Input: dimensioned drawing with shaded views. Units: mm. Origin: part minimum x, y, z. Coordinates: 2 decimals unless noted, no trailing zeros. Write each loop counter-clockwise with the first axis right and the second up, starting at its lowest first coordinate (ties: lowest second). Pieces come first, ordered by that corner, then holes. Notation, with made-up numbers: (35.5, 40) -> (73.5, 40) arc R23 ccw to (73.5, 69) -> close; hole circle Ø7 at (-31, -26.5). An arc over 180 degrees is marked (long way). One line per item, written item: value. Start each with the question number.
1. Section query A-A, the plane x = 7.5. Output: boundary loops of the cut face in (y, z).
2. Section query C-C, the plane z = 9.75. Output: boundary loops of the cut face in (x, y).
3. Line query: line 1 (Y direction, x = 7.5, z = 7); line 2 (Y direction, x = 10.5, z = 6.25); line 3 (X direction, y = 27, z = 5.25). Output: solid intervals per line, ascending.
4. Mould query, pull axis Y, two halves, no side actions, for the marked faces 1, 2 and 3. Classes: released by +Y, released by -Y, zero draft, split by the parting line, or undercut.
5. First-contact query: P1, Ø3, axis at x = 2.5, y = 25.5, coming from the -Z side; P2, Ø9, axis at x = 7.5, y = 30, coming from the -Z side. Flat tips, straight axial feed; report the tip coordinate or a pass-through.
6. Section query B-B, the plane y = 30. Output: boundary loops of the cut face in (x, z), and give its area (3 significant figures).
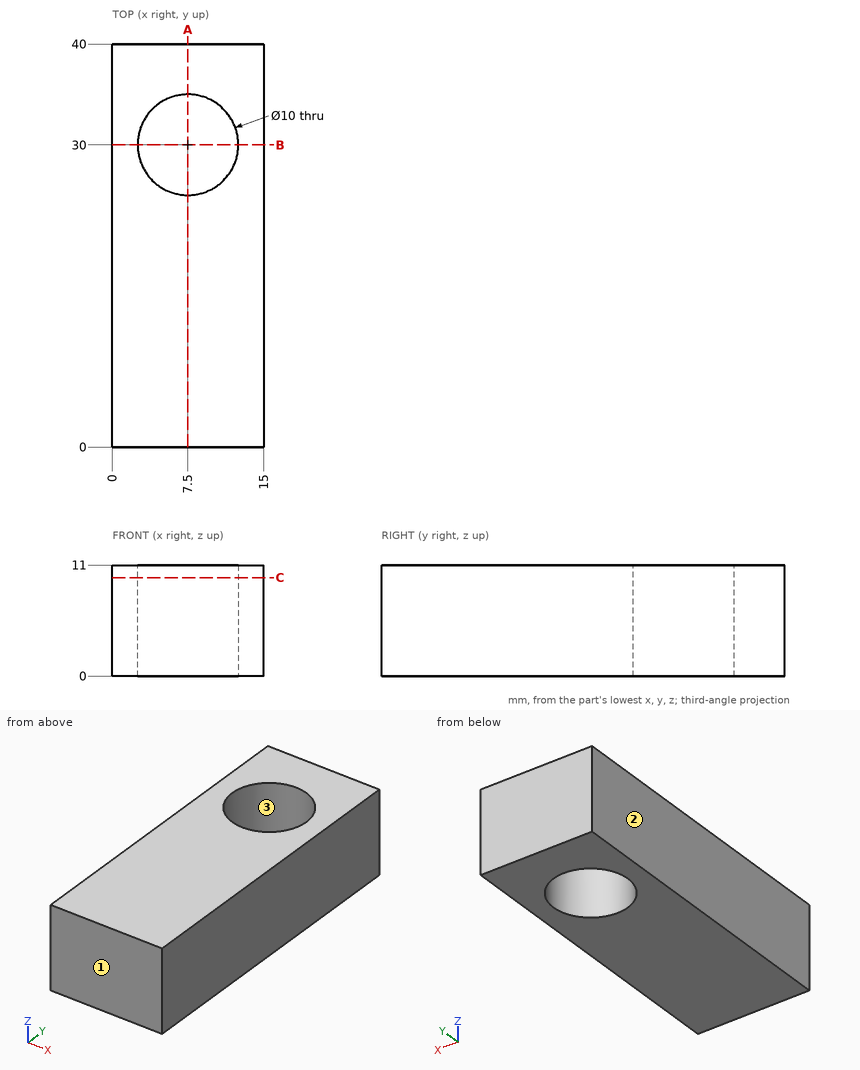
Computed values:
1. outline: (0, 0) -> (25, 0) -> (25, 11) -> (0, 11) -> close; (35, 0) -> (40, 0) -> (40, 11) -> (35, 11) -> close
2. outline: (0, 0) -> (15, 0) -> (15, 40) -> (0, 40) -> close; hole circle Ø10 at (7.5, 30)
3. line 1: y = 0 to 25, 35 to 40
3. line 2: y = 0 to 26, 34 to 40
3. line 3: x = 0 to 3.5, 11.5 to 15
4. face 1: released by -Y
4. face 2: zero draft
4. face 3: undercut
5. P1: stops at z = 0
5. P2: passes through
6. outline: (0, 0) -> (2.5, 0) -> (2.5, 11) -> (0, 11) -> close; (12.5, 0) -> (15, 0) -> (15, 11) -> (12.5, 11) -> close
6. area: 55.0 mm²
